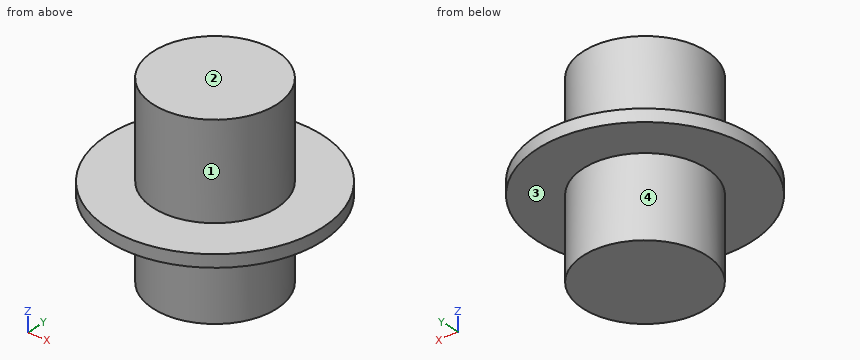
from build123d import *

# Parameters (mm, degrees)
CIRCLE001_R          = 8.697725
EXTRUDE_DEPTH        = 1
CYLINDER_R           = 5
CYLINDER_DEPTH       = 15
CLONE013_SCALE_SCALE = 2.2


with BuildPart() as obj1:
    # Circle001 → Extrude (new body)
    with BuildSketch(Plane.XY.offset(57.640399)):
        Circle(CIRCLE001_R)
    extrude(amount=EXTRUDE_DEPTH)


with BuildPart() as obj1_1:
    # Extrude placement: moved
    add(obj1.part.moved(Location((0, 0, -8.594981))))


with BuildPart() as obj2:
    # Cylinder → Cylinder (new body)
    with BuildSketch(Plane.XY.offset(42.640399)):
        Circle(CYLINDER_R)
    extrude(amount=CYLINDER_DEPTH)

    # Fusion002: union obj1
    add(obj1_1.part)


with BuildPart() as obj2_1:
    # Clone013 scale: moved
    add(obj2.part.scale(CLONE013_SCALE_SCALE))


solid = obj2_1.part
The model under review builds one solid part; all positions refer to its coordinate system, in mm. Face numbers are marked on the shaded views. A direction names the side the tool comes from. Round coordinates to 2 decimals unless told otherwise and drop trailing zeros. Order: outer loops, then holes, each group sorted by start corner. A loop starts at its lowest first (then second) coordinate and runs counter-clockwise, first axis right, second up. Notation, with made-up numbers: (64, -1) -> (97, -1) arc R12 ccw to (97, 22) -> close; hole circle Ø10 at (81, -15.75). An arc over 180 degrees is marked (long way). Use CSV: the item, a comma, the result in double quotes. Start each with the question number.
(1) Consider section D-D on y = 12. Write out the cut boundary in (x, z), and give its area (3 significant figures).
(2) Mouldability with a two-part tool opening along X and no side actions: class the marked faces 3 and 4 as pulls with the +X half, pulls with the -X half, needs draft (parallel to the pull), parting line crosses it, or undercut.
(3) Consider section A-A on y = 0. Write out the cut boundary in (x, z) (3 decimals).
(4) Consider section C-C on z = 120. Write out the cut boundary in (x, y).
(5) Tool access review of the marked faces 1 and 2: name each direction out of +Z, -Z, +X, -X, +Y, -Y from which nothing blocks a thin tool from reaching the whole face with its end or side.
(6) Insertion check: pin 1 (1.5 mm diameter, centred on x = -11, y = -11, fed in from -Z); pin 2 (8 mm diameter, centred on x = -13.5, y = 12.5, fed in from +Z); pin 3 (12 mm diameter, centred on x = -12.5, y = -0.5, fed in from -Z); pin 4 (3 mm diameter, centred on y = 4, z = 98.5, fed in from -X). Each pin has a flat end and moves straight along its axis. Give the tip position at first contact, or say it passes through.
(7) Wall thickness on probe 1 along Z at (x, y) = (6.5, 14.5); probe 2 along Y at (x, z) = (2, 111); probe 3 along X at (y, z) = (8, 117.5): over which ranges is each line inside the solid? List them lowest first. Write a range as from..to.
Responses:
1,outline,"(-14.9, 107.9) -> (14.9, 107.9) -> (14.9, 110.1) -> (-14.9, 110.1) -> close"
1,area,"65.6 mm²"
2,face 3,"needs draft"
2,face 4,"parting line crosses it"
3,outline,"(-19.135, 107.9) -> (-11, 107.9) -> (-11, 93.809) -> (11, 93.809) -> (11, 107.9) -> (19.135, 107.9) -> (19.135, 110.1) -> (11, 110.1) -> (11, 126.809) -> (-11, 126.809) -> (-11, 110.1) -> (-19.135, 110.1) -> close"
4,outline,"circle Ø22 at (0, 0)"
5,face 1,"+Z"
5,face 2,"+Z, +X, -X, +Y, -Y"
6,pin 1,"z = 107.9"
6,pin 2,"z = 110.1"
6,pin 3,"z = 93.81"
6,pin 4,"x = -10.71"
7,probe 1,"107.9..110.1"
7,probe 2,"-10.82..10.82"
7,probe 3,"-7.55..7.55"
